Check sheet for the drawn part. Datum: minimum x, y, z corner. Units: mm. A direction names the side the tool comes from. Give positions to 0.01 mm unless a question says otherwise; leave off trailing zeros. Order: outer loops, then holes, each group sorted by start corner. A loop starts at its lowest first (then second) coordinate and runs counter-clockwise, first axis right, second up. Notation, with made-up numbers: (-24, -26.5) - (27, -26.5) arc R19 ccw to (27, -10.5) - close; hole circle Ø2 at (-33, 6.25). An arc over 180 degrees is marked (long way). Answer as a JSON object with one key per item and string values. Group by question number.
(1) Mould release check, pull along X, two halves, no side actions. Record for the marked faces 3, 4 and 5: +X half, -X half, draft (parallel to the pull), parting line (faces both ways), or undercut.
(2) Section check A-A (x = 20). Record the boundary of the cut face in (y, z), then the cut area to 3 significant figures.
(3) Section check C-C (z = 3.25). Record the boundary of the cut face in (x, y), then the cut area to 3 significant figures.
(4) Access from +Z, -Z, +X, -X, +Y, -Y to the whole of each face (thin tool, end or side, straight path). Record for the marked faces 1 and 2.
(5) Depth check by flat-ended pin: pin 1 Ø9.5 at (x, y) = (27, 14.5) entering from +Z; pin 2 Ø1.5 at (x, z) = (28, 3.5) entering from -Y; pin 3 Ø4 at (x, z) = (28, 12.5) entering from +Y. Enter the tip coordinate at first touch or a pass-through.
(6) Thickness scan on line 1 (Y direction, x = 20, z = 15.2); line 2 (Y direction, x = 20, z = 17.75); line 3 (Z direction, x = 22.5, y = 29.5). Record the ranges inside material, lowest first.
(7) Section check D-D (z = 10). Record the boundary of the cut face in (x, y).
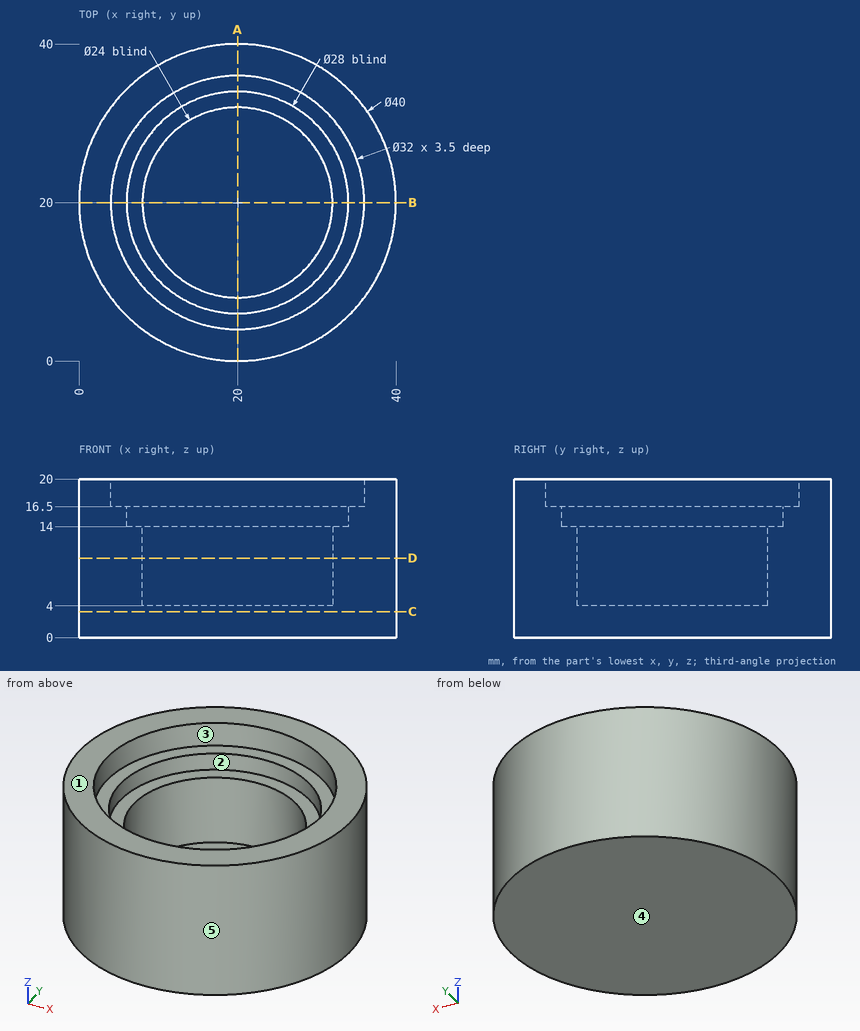
Solutions:
{
 "1": {"face 3": "undercut", "face 4": "draft", "face 5": "parting line"},
 "2": {"outline": "(0, 0) - (40, 0) - (40, 20) - (36, 20) - (36, 16.5) - (34, 16.5) - (34, 14) - (32, 14) - (32, 4) - (8, 4) - (8, 14) - (6, 14) - (6, 16.5) - (4, 16.5) - (4, 20) - (0, 20) - close", "area": "378 mm2"},
 "3": {"outline": "circle Ø40 at (20, 20)", "area": "1,260 mm2"},
 "4": {"face 1": "+Z, +X, -X, +Y, -Y", "face 2": "+Z"},
 "5": {"pin 1": "stops at z = 14", "pin 2": "stops at y = 1.36", "pin 3": "stops at y = 39.08"},
 "6": {"line 1": "y = 0 to 6, 34 to 40", "line 2": "y = 0 to 4, 36 to 40", "line 3": "z = 0 to 4"},
 "7": {"outline": "circle Ø40 at (20, 20); hole circle Ø24 at (20, 20)"}
}
